Autodesk Inventor part; units mm, degrees
ref_plane "РабПлоскость1" through (0, -4, 0) normal (0, 1, 0) x (-1, 0, 0)
ref_plane "YZ Plane" through (0, 0, 0) normal (1, 0, 0) x (0, 1, 0)
ref_plane "XY Plane" through (0, 0, 0) normal (0, 0, 1) x (1, 0, 0)
sketch "Эскиз1" plane through (0, 0, 0) normal (1, 0, 0) x (0, 1, 0)
  circle A0 centre (0, 0) radius 1.5
  circle A1 centre (0, 0) radius 4
  dimension "d0" = 3
  dimension "d1" = 8
extrude "Выдавливание1" add sketch "Эскиз1" along normal blind 12
sketch "Эскиз2" plane through (12, 0, 0) normal (1, 0, 0) x (0, 0, -1)
  circle A0 centre (0, 0) radius 1.5
  circle A1 centre (0, 0) radius 4
  circle A2 centre (0, 0) radius 2.5
  dimension "d4" = 5
extrude "Выдавливание2" add sketch "Эскиз2" along normal blind 4 contours A2
ref_plane "РабПлоскость1" through (0, -4, 0) normal (0, 1, 0) x (-1, 0, 0)
sketch "Эскиз3" plane through (0, -4, 0) normal (0, 1, 0) x (-1, 0, 0)
  point P0 (0, 0)
  point P1 (-3, 0)
  point P2 (-9, 0)
  dimension "d7" = 3
  dimension "d8" = 6
hole "Отверстие1" at (3, -4, 0) at (9, -4, 0) direction (0, 1, 0) diameter 2.459 depth 3 tip angle 118
properties part number "Vtulka"
Geometry: final body of the model. Coordinates: model frame, mm. A direction names the side the tool comes from. Give positions to 0.01 mm unless a question says otherwise; leave off trailing zeros. Order: outer loops, then holes, each group sorted by start corner. A loop starts at its lowest first (then second) coordinate and runs counter-clockwise, first axis right, second up. Notation, with made-up numbers: (-11.5, 50) - (10.5, 50) arc R14 ccw to (10.5, 69) - close; hole circle Ø8 at (0.5, 79.5). An arc over 180 degrees is marked (long way). Use CSV: the item, a comma, the result in double quotes.
1. Section query A-A (z = 0). Output: boundary loops of the cut face in (x, y).
Answers below:
outline,"(0, -4) - (1.77, -4) - (1.77, -1.5) - (0, -1.5) - close; (0, 1.5) - (16, 1.5) - (16, 2.5) - (12, 2.5) - (12, 4) - (0, 4) - close; (4.23, -4) - (7.77, -4) - (7.77, -1.5) - (4.23, -1.5) - close; (10.23, -4) - (12, -4) - (12, -2.5) - (16, -2.5) - (16, -1.5) - (10.23, -1.5) - close"
2. Section query B-B (y = 0). Output: boundary loops of the cut face in (x, z), plus the area to 3 significant figures.
Answers below:
outline,"(0, -4) - (12, -4) - (12, -2.5) - (16, -2.5) - (16, -1.5) - (0, -1.5) - close; (0, 1.5) - (16, 1.5) - (16, 2.5) - (12, 2.5) - (12, 4) - (0, 4) - close"
area,"68.0 mm2"
3. Mould query, pull axis Z, two halves, no side actions, for faces 1 (the face through (7.89, 1.39, -0.56)), 2 (the face through (13.97, 2.44, 0.54)), 3 (the face through (12, 2, 2)). Classes: +Z half, -Z half, draft (parallel to the pull), parting line (faces both ways), or undercut.
Answers below:
face 1,"undercut"
face 2,"parting line"
face 3,"draft"
4. Section query C-C (x = 14.75). Output: boundary loops of the cut face in (y, z), plus the area to 3 significant figures.
Answers below:
outline,"circle Ø5 at (0, 0); hole circle Ø3 at (0, 0)"
area,"12.6 mm2"
5. Material intervals for line 1 along Y through (x, z) = (13.25, 0); line 2 along Z through (x, y) = (7.25, 0); line 3 along X through (y, z) = (-1.5, 3.5), sorted ascending. Write a range as from..to.
Answers below:
line 1,"-2.5..-1.5, 1.5..2.5"
line 2,"-4..-1.5, 1.5..4"
line 3,"0..12"
6. Access query for faces 4 (the face through (4.09, -2.48, -0.57)), 5 (the face through (0, 2, 0)). Directions: +Z, -Z, +X, -X, +Y, -Y. A direction counts if a zero-diameter tool reaches every point of the face in a straight line with its end or side. Return the directions, or none.
Answers below:
face 4,"-Y"
face 5,"+Z, -Z, -X, +Y, -Y"
7. Section query D-D (y = -3.5). Output: boundary loops of the cut face in (x, z), plus the area to 3 significant figures.
Answers below:
outline,"(0, -1.94) - (12, -1.94) - (12, 1.94) - (0, 1.94) - close; hole circle Ø2.46 at (3, 0); hole circle Ø2.46 at (9, 0)"
area,"37.0 mm2"
8. Contact query for flat-ended pins moving along their axis: pin 1 (1 mm diameter, centred on x = 10.5, y = -2, fed in from -Z); pin 2 (1.5 mm diameter, centred on x = 3, z = 0, fed in from -Y); pin 3 (2 mm diameter, centred on x = 7, y = 3, fed in from -Z). Output: stop coordinate, or through.
Answers below:
pin 1,"z = -3.71"
pin 2,"y = 1.3"
pin 3,"z = -3.46"
